Autodesk Inventor part; units mm, degrees
ref_plane "YZ Plane" through (0, 0, 0) normal (1, 0, 0) x (0, 1, 0)
ref_plane "XZ Plane" through (0, 0, 0) normal (0, 1, 0) x (-1, 0, 0)
ref_plane "XY Plane" through (0, 0, 0) normal (0, 0, 1) x (1, 0, 0)
sketch "Esboço1" plane through (0, 0, 0) normal (1, 0, 0) x (0, 1, 0)
  arc A0 (24.6347, 5.5491) -> (24.6347, -0.4509) centre (12.5, 2.5491) ccw
  line L0 (34, 2.5491) -> (34, 17.5491)
  line L1 (34, 2.5491) -> (34, -12.4509)
  line L2 (31, 5.5491) -> (24.6347, 5.5491)
  line L3 (31, -0.4509) -> (24.6347, -0.4509)
  line L4 (31, 17.5491) -> (31, 5.5491)
  line L5 (31, -0.4509) -> (31, -12.4509)
  line L6 (34, 17.5491) -> (34, 22.5491)
  line L7 (31, 17.5491) -> (31, 22.5491)
  line L8 (31, 22.5491) -> (34, 22.5491)
  line L9 (34, -12.4509) -> (34, -17.4509)
  line L10 (34, -17.4509) -> (31, -17.4509)
  line L11 (31, -17.4509) -> (31, -12.4509)
  point P0 (0, 0)
  dimension "d2" = 25
  dimension "d4" = 15
  dimension "d7" = 3
  dimension "d10" = 5
  dimension "d11" = 5
extrude "Extrusão2" add sketch "Esboço1" along normal blind 34
properties part number "boba"
Geometry check sheet. Reference: the model listing, model coordinates, mm. A direction names the side the tool comes from. Coordinates: 2 decimals unless noted, no trailing zeros. Order: outer loops, then holes, each group sorted by start corner. A loop starts at its lowest first (then second) coordinate and runs counter-clockwise, first axis right, second up.
Q1. Tool access check on faces 5 (the face through (0, 17, 3)), 6 (the face through (17, 28, -0.451)), 7 (the face through (17, 28, 5.549)). Record the directions out of +Z, -Z, +X, -X, +Y, -Y that give a thin tool (end or side, any length) a straight path to the whole face; none if there is none.
Reply:
face 5: +Z, -Z, -X, +Y, -Y
face 6: -Z, +X, -X
face 7: +Z, +X, -X
Q2. Sectioned sample at C-C on y = 12.5. Record the cut outline in (x, z), and give its area (3 significant figures).
Reply:
outline: (0, -9.95) - (34, -9.95) - (34, 15.05) - (0, 15.05) - close
area: 850 mm2
Q3. Sectioned sample at A-A on z = -3.5. Record the cut outline in (x, y).
Reply:
outline: (0, 1.56) - (34, 1.56) - (34, 23.44) - (0, 23.44) - close; (0, 31) - (34, 31) - (34, 34) - (0, 34) - close
Q4. Draft check along Y on faces 1 (the face through (17, 33, -17.451)), 2 (the face through (17, 31, 14)), 3 (the face through (17, 31, -9)), 4 (the face through (17, 34, 2)). Enter one of: released by +Y, released by -Y, zero draft, split by the parting line, or undercut.
Reply:
face 1: zero draft
face 2: undercut
face 3: undercut
face 4: released by +Y
Q5. Depth check by flat-ended pin: pin 1 Ø6 at (y, z) = (4, 17) entering from -X; pin 2 Ø4 at (x, y) = (10.5, 5.5) entering from -Z; pin 3 Ø8.5 at (x, z) = (9, 18) entering from -Y; pin 4 Ø5 at (x, y) = (13.5, 26.5) entering from +Z. Enter the tip coordinate at first touch or a pass-through.
Reply:
pin 1: passes through
pin 2: stops at z = -8.91
pin 3: stops at y = 6.95
pin 4: stops at z = 7.45
Q6. Sectioned sample at D-D on z = 18.5. Record the cut outline in (x, y), and give its area (3 significant figures).
Reply:
outline: (0, 31) - (34, 31) - (34, 34) - (0, 34) - close
area: 102 mm2
Q7. Thickness scan on probe 1 along Y at (x, z) = (26, -4.5); probe 2 along Y at (x, z) = (20, -2.5); probe 3 along Y at (x, z) = (11, 17). Record the ranges inside material, lowest first.
Reply:
probe 1: y = 2.18 to 22.82, 31 to 34
probe 2: y = 1.07 to 23.93, 31 to 34
probe 3: y = 31 to 34
Q8. Sectioned sample at B-B on x = 17. Record the cut outline in (y, z).
Reply:
outline: (24.63, -0.45) - (31, -0.45) - (31, -17.45) - (34, -17.45) - (34, 22.55) - (31, 22.55) - (31, 5.55) - (24.63, 5.55) arc R12.5 ccw (long way) to start
